Geometry: see drawing. Coordinates: mm, zero at the bounding-box minimum. A direction names the side the tool comes from. Give positions to 0.01 mm unless a question says otherwise; leave off trailing zeros. Order: outer loops, then holes, each group sorted by start corner. A loop starts at its lowest first (then second) coordinate and runs counter-clockwise, first axis right, second up. Notation, with made-up numbers: M 24.25,-18 L 43.25,-18 A7 cw 43.25,-8 Z; hole C -25.5,35 d2. An arc over 180 degrees is marked long. Write item = value, one per line. Start each with the question number.
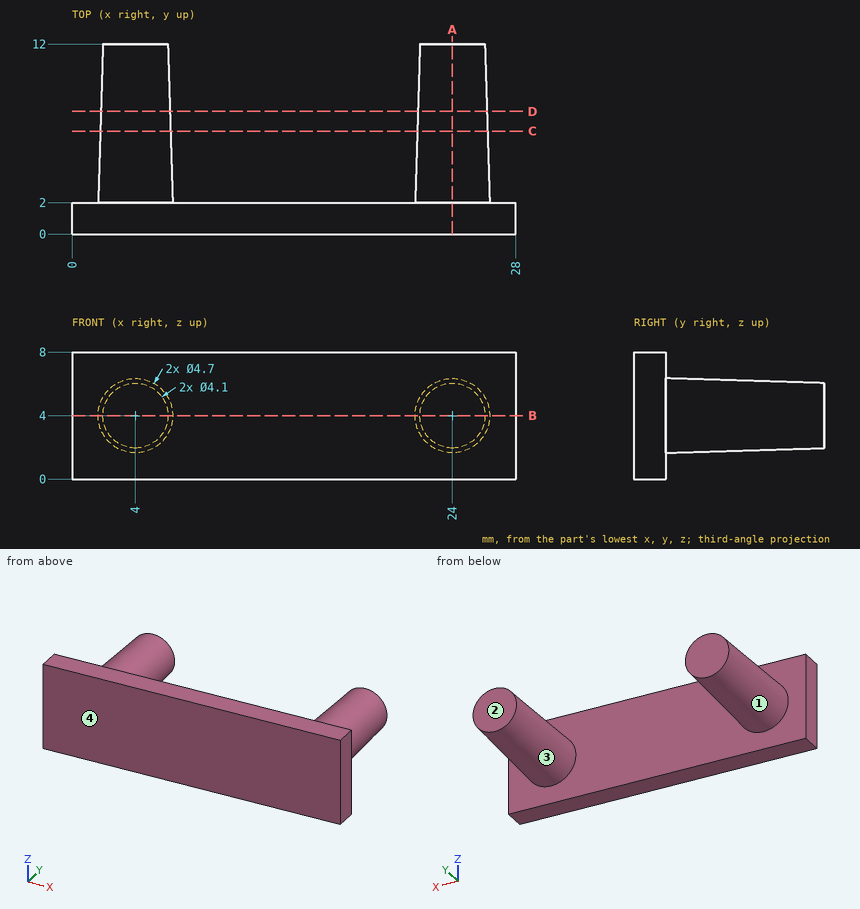
1) Cut plane B-B (z = 4). Return loops of the section in (x, y).
2) Cut plane D-D (y = 7.75). Return loops of the section in (x, z) (1 decimal).
3) Ray query, L1, parallel to Y at x = 7, z = 4; L2, parallel to X at y = 2.75, z = 2.25; L3, parallel to X at y = 8.5, z = 4.25. Return the intervals inside material, ascending.
4) Cut plane C-C (y = 6.5). Return loops of the section in (x, z) (3 decimals).
5) Cut plane A-A (x = 24). Return loops of the section in (y, z), plus the area to 3 significant figures.
6) Access query for the marked faces 3 and 4. Directions: +Z, -Z, +X, -X, +Y, -Y. A direction counts if a zero-diameter tool reaches every point of the face in a straight line with its end or side. Return the directions, or none.
7) Pin query (flat end, axial travel): pin 1 Ø3 at (y, z) = (10.5, 4) entering from +X; pin 2 Ø1.5 at (y, z) = (3, 6) entering from +X; pin 3 Ø1 at (x, z) = (17, 6) entering from +Y. Return the tip coordinate at first contact, or that it passes through.
8) Draft query along X for the marked faces 1 and 2. Return one class per face: pulls with the +X half, pulls with the -X half, needs draft (parallel to the pull), parting line crosses it, or undercut.
Reply:
q1.outline = M 0,0 L 28,0 L 28,2 L 26.35,2 L 26.05,12 L 21.95,12 L 21.65,2 L 6.35,2 L 6.05,12 L 1.95,12 L 1.65,2 L 0,2 Z
q2.outline = C 4,4 d4.4; C 24,4 d4.4
q3.L1 = 0 to 2
q3.L2 = 2.47 to 5.53, 22.47 to 25.53
q3.L3 = 1.86 to 6.14, 21.86 to 26.14
q4.outline = C 4,4 d4.43; C 24,4 d4.43
q5.outline = M 0,0 L 2,0 L 2,1.65 L 12,1.95 L 12,6.05 L 2,6.35 L 2,8 L 0,8 Z
q5.area = 60.0 mm²
q6.face_3 = +Y
q6.face_4 = +Z, -Z, +X, -X, -Y
q7.pin_1 = 26.14
q7.pin_2 = 25.96
q7.pin_3 = 2
q8.face_1 = undercut
q8.face_2 = needs draft
